Can you work these out from the drawing? Everything is in mm from the part's minimum corner. A direction names the side the tool comes from. Round coordinates to 2 decimals unless told otherwise and drop trailing zeros. Write each loop counter-clockwise with the first axis right and the second up, starting at its lowest first coordinate (ties: lowest second). Pieces come first, ordered by that corner, then holes. Notation, with made-up numbers: M 25.5,-28 L 43.5,-28 A30 cw 43.5,11 Z; hole C 37,86.5 d1. An arc over 180 degrees is marked long. Use a Markdown table: item, result. Add a question column.
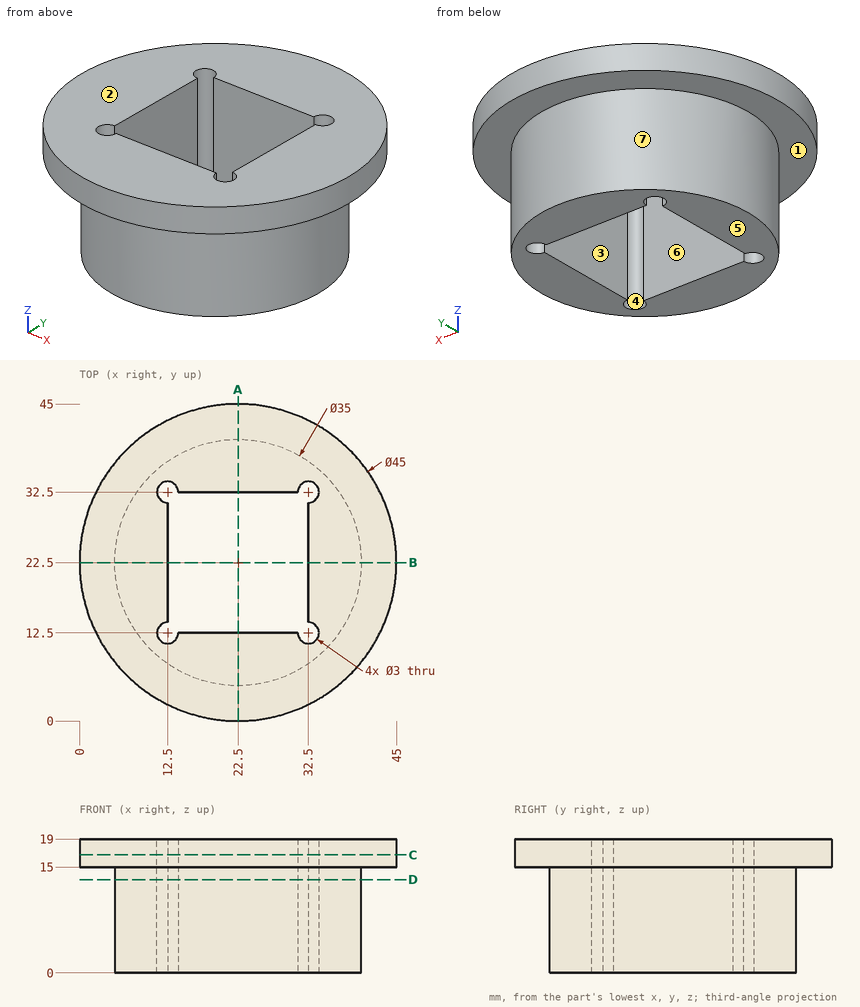
Item 1: Imagine slicing it at D-D on z = 13.25. List the corners of the cut face in (x, y) for me.
Item 2: For pin 1 Ø3 at (y, z) = (12, 9) entering from +X; pin 2 Ø5 at (y, z) = (21, 11) entering from +X; pin 3 Ø5 at (x, z) = (36.5, 10.5) entering from +Y; pin 4 Ø4 at (x, y) = (16.5, 29) entering from -Z, each with a flat end and sliding along its axis, tell me the tip position at first contact or that it passes through.
Item 3: On a 3-axis mill with a long thin cutter (end or side, diameter ignored), from which of +Z, -Z, +X, -X, +Y, -Y can I reach the whole of each face in a straight line? I mean the marked faces 1, 2 and 3. Say none if no direction works.
Item 4: Imagine slicing it at A-A on x = 22.5. List the corners of the cut face in (y, z) for me, plus the area to 3 significant figures.
Item 5: If we mould it in two halves opening along X, with no side actions, what happens to the marked faces 4, 5, 6 and 7? For each: +X half, -X half, draft (parallel to the pull), parting line (faces both ways), or undercut.
Item 6: I need wall thicknesses on probe 1 along Y at (x, z) = (33, 17.75); probe 2 along X at (y, z) = (33, 13.5); probe 3 along Y at (x, z) = (21.5, 3.5). Which ranges of each line are inside material? Lowest first, please. Write a range as from..to.
Item 7: Imagine slicing it at C-C on z = 16.75. List the corners of the cut face in (x, y) for me.
The answers:
| question | item | result |
|---|---|---|
| 1 | outline | C 22.5,22.5 d35; hole M 12.5,14 A1.5 ccw long 14,12.5 L 31,12.5 A1.5 ccw long 32.5,14 L 32.5,31 A1.5 ccw long 31,32.5 L 14,32.5 A1.5 ccw long 12.5,31 Z |
| 2 | pin 1 | x = 37.51 |
| 2 | pin 2 | x = 40 |
| 2 | pin 3 | y = 35.69 |
| 2 | pin 4 | through |
| 3 | face 1 | -Z |
| 3 | face 2 | +Z, +X, -X, +Y, -Y |
| 3 | face 3 | +Z, -Z |
| 4 | outline | M 0,15 L 5,15 L 5,0 L 12.5,0 L 12.5,19 L 0,19 Z; M 32.5,0 L 40,0 L 40,15 L 45,15 L 45,19 L 32.5,19 Z |
| 4 | area | 325 mm² |
| 5 | face 4 | undercut |
| 5 | face 5 | draft |
| 5 | face 6 | undercut |
| 5 | face 7 | parting line |
| 6 | probe 1 | 2.6..11.09, 13.91..31.09, 33.91..42.4 |
| 6 | probe 2 | 8.5..11.09, 13.91..31.09, 33.91..36.5 |
| 6 | probe 3 | 5.03..12.5, 32.5..39.97 |
| 7 | outline | C 22.5,22.5 d45; hole M 12.5,14 A1.5 ccw long 14,12.5 L 31,12.5 A1.5 ccw long 32.5,14 L 32.5,31 A1.5 ccw long 31,32.5 L 14,32.5 A1.5 ccw long 12.5,31 Z |
